Here's how the part is built. I have some questions about the finished solid (model axes, mm). Coordinates: 2 decimals unless noted, no trailing zeros. Write each loop counter-clockwise with the first axis right and the second up, starting at its lowest first coordinate (ties: lowest second). Pieces come first, ordered by that corner, then holes. Notation, with made-up numbers: (19, 85.5) -> (44, 85.5) arc R31 ccw to (44, 116.5) -> close; hole circle Ø9 at (52, 21). An arc over 180 degrees is marked (long way). Use a Markdown table: item, result. Add a question column.
Item 1: Imagine slicing it at B-B, the plane z = 3.7. Count the separate pieces of the cut face and the enclosed holes in it, and give its area (3 significant figures).
Item 2: Will this pin go through, and if not, where does the flat tip stop? pin 1 Ø15 at (x, y) = (-108.63, 0) entering from -Z.
Item 3: If we mould it in two halves opening along Y, with no side actions, what happens to faces 1 (the cylindrical face through (85.176, 1.824, 2.348)), 2 (the flat face through (-2, 0, 4.762)), 3 (the flat face through (-2, 19.05, 2))? For each: pulls with the +Y half, pulls with the -Y half, needs draft (parallel to the pull), parting line crosses it, or undercut.
Item 4: Imagine slicing it at A-A, the plane y = 0. Write out the boundary of the cut face in (x, z), and give its area (3 significant figures).
```python
from build123d import *

# Parameters (mm, degrees)
SKETCH1_W           = 241.3
SKETCH1_H           = 38.1
SKETCH1_R           = 4.7625
BOSS_EXTRUDE1_DEPTH = 4.7625


with BuildPart() as part:
    # Sketch1 → Boss-Extrude1 (new body)
    with BuildSketch(Plane.XY):
        Rectangle(SKETCH1_W, SKETCH1_H)
        with Locations(Location((-108.625531915, 0, 0), (0, 0, 180))):
            Circle(SKETCH1_R, mode=Mode.SUBTRACT)
        with Locations(Location((-89.575531915, 0, 0), (0, 0, 180))):
            Circle(SKETCH1_R, mode=Mode.SUBTRACT)
        with Locations(Location((89.575531915, 0, 0), (0, 0, 180))):
            Circle(SKETCH1_R, mode=Mode.SUBTRACT)
        with Locations(Location((108.625531915, 0, 0), (0, 0, 180))):
            Circle(SKETCH1_R, mode=Mode.SUBTRACT)
    extrude(amount=BOSS_EXTRUDE1_DEPTH)


solid = part.part
```
Ans:
| question | item | result |
|---|---|---|
| 1 | separate pieces | 1 |
| 1 | enclosed holes | 4 |
| 1 | area | 8,910 mm^2 |
| 2 | pin 1 | stops at z = 0 |
| 3 | face 1 | undercut |
| 3 | face 2 | needs draft |
| 3 | face 3 | pulls with the +Y half |
| 4 | outline | (-120.65, 0) -> (-113.39, 0) -> (-113.39, 4.76) -> (-120.65, 4.76) -> close; (-103.86, 0) -> (-94.34, 0) -> (-94.34, 4.76) -> (-103.86, 4.76) -> close; (-84.81, 0) -> (84.81, 0) -> (84.81, 4.76) -> (-84.81, 4.76) -> close; (94.34, 0) -> (103.86, 0) -> (103.86, 4.76) -> (94.34, 4.76) -> close; (113.39, 0) -> (120.65, 0) -> (120.65, 4.76) -> (113.39, 4.76) -> close |
| 4 | area | 968 mm^2 |
